Build history of the part. All positions in model axes, mm. A direction names the side the tool comes from. Round coordinates to 2 decimals unless told otherwise and drop trailing zeros. Write each loop counter-clockwise with the first axis right and the second up, starting at its lowest first coordinate (ties: lowest second). Pieces come first, ordered by that corner, then holes. Notation, with made-up numbers: M -9,60 L 14,60 A25 cw 14,96 Z; hole C -13,16 d7. An arc over 180 degrees is marked long. Write item = value, one per line.
from build123d import *

# Parameters (mm, degrees)
SKETCH1_R           = 1.7
BOSS_EXTRUDE1_DEPTH = 5
CUT_EXTRUDE1_DEPTH  = 2
SKETCH3_R           = 3
CUT_EXTRUDE2_DEPTH  = 2
SKETCH4_R           = 1.9
CUT_EXTRUDE3_DEPTH  = 3
SKETCH5_R           = 0.8
CUT_EXTRUDE4_DEPTH  = 3
CUT_EXTRUDE8_DEPTH  = 0.8
FILLET1_R           = 1.5875
CUT_EXTRUDE9_REACH  = 64.803
SKETCH8_W           = 7.193942136
SKETCH8_H           = 8.27
FILLET2_R           = 1.5875
SKETCH9_W           = 5
SKETCH9_H           = 0.25
CUT_EXTRUDE11_DEPTH = 5


with BuildPart() as part:
    # Sketch1 → Boss-Extrude1 (new body)
    with BuildSketch(Plane.XY):
        with BuildLine():
            Line((43, -3.052490593), (43, 3.052490593))
            ThreePointArc((43, 3.052490593), (42.8123201, 3.635702437), (42.319727891, 4))
            ThreePointArc((42.319727891, 4), (39.191767362, 6.313289526), (38, 10.016684732))
            Line((38, 10.016684732), (38, 24.575474703))
            ThreePointArc((38, 24.575474703), (38.684894673, 27.444112294), (40.591836735, 29.693942136))
            ThreePointArc((40.591836735, 29.693942136), (40.892142571, 30.048246049), (41, 30.5))
            Line((41, 30.5), (41, 35.5))
            Line((41, 35.5), (34, 35.5))
            ThreePointArc((34, 35.5), (33.292893219, 35.792893219), (33, 36.5))
            Line((33, 36.5), (33, 43.5))
            Line((33, 43.5), (28, 43.5))
            ThreePointArc((28, 43.5), (27.548246049, 43.392142571), (27.193942136, 43.091836735))
            ThreePointArc((27.193942136, 43.091836735), (24.944112294, 41.184894673), (22.075474703, 40.5))
            Line((22.075474703, 40.5), (10.016684732, 40.5))
            ThreePointArc((10.016684732, 40.5), (6.313289526, 41.691767362), (4, 44.819727891))
            ThreePointArc((4, 44.819727891), (3.635702437, 45.3123201), (3.052490593, 45.5))
            Line((3.052490593, 45.5), (-3.052490593, 45.5))
            ThreePointArc((-3.052490593, 45.5), (-3.635702437, 45.3123201), (-4, 44.819727891))
            ThreePointArc((-4, 44.819727891), (-6.313289526, 41.691767362), (-10.016684732, 40.5))
            Line((-10.016684732, 40.5), (-27.881532566, 40.5))
            ThreePointArc((-27.881532566, 40.5), (-30.750170158, 41.184894673), (-33, 43.091836735))
            ThreePointArc((-33, 43.091836735), (-33.354303912, 43.392142571), (-33.806057864, 43.5))
            Line((-33.806057864, 43.5), (-40, 43.5))
            ThreePointArc((-40, 43.5), (-40.707106781, 43.207106781), (-41, 42.5))
            Line((-41, 42.5), (-41, 36.306057864))
            ThreePointArc((-41, 36.306057864), (-40.892142571, 35.854303912), (-40.591836735, 35.5))
            ThreePointArc((-40.591836735, 35.5), (-38.684894673, 33.250170158), (-38, 30.381532566))
            Line((-38, 30.381532566), (-38, 10.016684732))
            ThreePointArc((-38, 10.016684732), (-39.191767362, 6.313289526), (-42.319727891, 4))
            ThreePointArc((-42.319727891, 4), (-42.8123201, 3.635702437), (-43, 3.052490593))
            Line((-43, 3.052490593), (-43, -3.052490593))
            ThreePointArc((-43, -3.052490593), (-42.8123201, -3.635702437), (-42.319727891, -4))
            ThreePointArc((-42.319727891, -4), (-39.191767362, -6.313289526), (-38, -10.016684732))
            Line((-38, -10.016684732), (-38, -30.381532566))
            ThreePointArc((-38, -30.381532566), (-38.684894673, -33.250170158), (-40.591836735, -35.5))
            ThreePointArc((-40.591836735, -35.5), (-40.892142571, -35.854303912), (-41, -36.306057864))
            Line((-41, -36.306057864), (-41, -42.5))
            ThreePointArc((-41, -42.5), (-40.707106781, -43.207106781), (-40, -43.5))
            Line((-40, -43.5), (-33.806057864, -43.5))
            ThreePointArc((-33.806057864, -43.5), (-33.354303912, -43.392142571), (-33, -43.091836735))
            ThreePointArc((-33, -43.091836735), (-30.750170158, -41.184894673), (-27.881532566, -40.5))
            Line((-27.881532566, -40.5), (-10.016684732, -40.5))
            ThreePointArc((-10.016684732, -40.5), (-6.313289526, -41.691767362), (-4, -44.819727891))
            ThreePointArc((-4, -44.819727891), (-3.635702437, -45.3123201), (-3.052490593, -45.5))
            Line((-3.052490593, -45.5), (3.052490593, -45.5))
            ThreePointArc((3.052490593, -45.5), (3.635702437, -45.3123201), (4, -44.819727891))
            ThreePointArc((4, -44.819727891), (6.313289526, -41.691767362), (10.016684732, -40.5))
            Line((10.016684732, -40.5), (27.881532566, -40.5))
            ThreePointArc((27.881532566, -40.5), (30.750170158, -41.184894673), (33, -43.091836735))
            ThreePointArc((33, -43.091836735), (33.354303912, -43.392142571), (33.806057864, -43.5))
            Line((33.806057864, -43.5), (40, -43.5))
            ThreePointArc((40, -43.5), (40.707106781, -43.207106781), (41, -42.5))
            Line((41, -42.5), (41, -36.306057864))
            ThreePointArc((41, -36.306057864), (40.892142571, -35.854303912), (40.591836735, -35.5))
            ThreePointArc((40.591836735, -35.5), (38.684894673, -33.250170158), (38, -30.381532566))
            Line((38, -30.381532566), (38, -10.016684732))
            ThreePointArc((38, -10.016684732), (39.191767362, -6.313289526), (42.319727891, -4))
            ThreePointArc((42.319727891, -4), (42.8123201, -3.635702437), (43, -3.052490593))
        make_face()
        with Locations((0, -42.5)):
            Circle(SKETCH1_R, mode=Mode.SUBTRACT)
        with Locations((-40, 0)):
            Circle(SKETCH1_R, mode=Mode.SUBTRACT)
        with Locations((40, 0)):
            Circle(SKETCH1_R, mode=Mode.SUBTRACT)
        with Locations((0, 42.5)):
            Circle(SKETCH1_R, mode=Mode.SUBTRACT)
        with Locations((38, 32.5)):
            Circle(SKETCH1_R, mode=Mode.SUBTRACT)
        with Locations((30, 40.5)):
            Circle(SKETCH1_R, mode=Mode.SUBTRACT)
    extrude(amount=-BOSS_EXTRUDE1_DEPTH)

    # Sketch2 → Cut-Extrude1 (cut)
    with BuildSketch(Plane(origin=(0, 0, -5), x_dir=(-1, 0, 0), z_dir=(0, 0, -1))):
        with BuildLine():
            Line((-20, 37.5), (20, 37.5))
            ThreePointArc((20, 37.5), (30.606601718, 33.106601718), (35, 22.5))
            Line((35, 22.5), (35, -22.5))
            ThreePointArc((35, -22.5), (30.606601718, -33.106601718), (20, -37.5))
            Line((20, -37.5), (-20, -37.5))
            ThreePointArc((-20, -37.5), (-30.606601718, -33.106601718), (-35, -22.5))
            Line((-35, -22.5), (-35, 22.5))
            ThreePointArc((-35, 22.5), (-30.606601718, 33.106601718), (-20, 37.5))
        make_face()
    extrude(amount=-CUT_EXTRUDE1_DEPTH, mode=Mode.SUBTRACT)

    # Sketch3 → Cut-Extrude2 (cut)
    with BuildSketch(Plane.XY):
        with Locations((-37, 39.5)):
            Circle(SKETCH3_R)
        with Locations((-37, -39.5)):
            Circle(SKETCH3_R)
        with Locations((37, -39.5)):
            Circle(SKETCH3_R)
        with BuildLine():
            Line((40, 3), (43, 3))
            Line((43, 3), (43, -3))
            Line((43, -3), (40, -3))
            ThreePointArc((40, -3), (37, 0), (40, 3))
        make_face()
        with BuildLine():
            Line((-40, 3), (-43, 3))
            Line((-43, 3), (-43, -3))
            Line((-43, -3), (-40, -3))
            ThreePointArc((-40, -3), (-37, 0), (-40, 3))
        make_face()
        with BuildLine():
            Line((-3, 42.5), (-3, 45.5))
            Line((-3, 45.5), (3, 45.5))
            Line((3, 45.5), (3, 42.5))
            ThreePointArc((3, 42.5), (0, 39.5), (-3, 42.5))
        make_face()
        with BuildLine():
            Line((-3, -42.5), (-3, -45.5))
            Line((-3, -45.5), (3, -45.5))
            Line((3, -45.5), (3, -42.5))
            ThreePointArc((3, -42.5), (0, -39.5), (-3, -42.5))
        make_face()
        with BuildLine():
            Line((38, 29.5), (40.341066152, 29.5))
            ThreePointArc((40.341066152, 29.5), (40.465240963, 29.598536241), (40.591836735, 29.693942136))
            ThreePointArc((40.591836735, 29.693942136), (40.892142571, 30.048246049), (41, 30.5))
            Line((41, 30.5), (41, 35.5))
            Line((41, 35.5), (35, 35.5))
            Line((35, 35.5), (35, 32.5))
            ThreePointArc((35, 32.5), (35.878679656, 30.378679656), (38, 29.5))
        make_face()
        with BuildLine():
            Line((30, 37.5), (33, 37.5))
            Line((33, 37.5), (33, 43.5))
            Line((33, 43.5), (28, 43.5))
            ThreePointArc((28, 43.5), (27.548246049, 43.392142571), (27.193942136, 43.091836735))
            ThreePointArc((27.193942136, 43.091836735), (27.098536241, 42.965240963), (27, 42.841066152))
            Line((27, 42.841066152), (27, 40.5))
            ThreePointArc((27, 40.5), (27.878679656, 38.378679656), (30, 37.5))
        make_face()
    extrude(amount=-CUT_EXTRUDE2_DEPTH, mode=Mode.SUBTRACT)

    # Sketch4 → Cut-Extrude3 (cut)
    with BuildSketch(Plane.XY.offset(-2)):
        with Locations((-37, 39.5)):
            Circle(SKETCH4_R)
        with Locations((37, -39.5)):
            Circle(SKETCH4_R)
        with Locations((-37, -39.5)):
            Circle(SKETCH4_R)
    extrude(amount=-CUT_EXTRUDE3_DEPTH, mode=Mode.SUBTRACT)

    # Sketch5 → Cut-Extrude4 (cut)
    with BuildSketch(Plane.XY):
        with Locations((-17.109, -19.609)):
            Circle(SKETCH5_R)
        with Locations((-14.109, -19.609)):
            Circle(SKETCH5_R)
        with Locations((-11.109, -19.609)):
            Circle(SKETCH5_R)
        with Locations((-8.109, -19.609)):
            Circle(SKETCH5_R)
        with Locations((-17.109, -22.609)):
            Circle(SKETCH5_R)
        with Locations((-14.109, -22.609)):
            Circle(SKETCH5_R)
        with Locations((-11.109, -22.609)):
            Circle(SKETCH5_R)
        with Locations((-8.109, -22.609)):
            Circle(SKETCH5_R)
        with Locations((-17.109, -25.609)):
            Circle(SKETCH5_R)
        with Locations((-14.109, -25.609)):
            Circle(SKETCH5_R)
        with Locations((-11.109, -25.609)):
            Circle(SKETCH5_R)
        with Locations((-8.109, -25.609)):
            Circle(SKETCH5_R)
        with Locations((-17.109, -16.609)):
            Circle(SKETCH5_R)
        with Locations((-14.109, -16.609)):
            Circle(SKETCH5_R)
        with Locations((-11.109, -16.609)):
            Circle(SKETCH5_R)
        with Locations((-8.109, -16.609)):
            Circle(SKETCH5_R)
    extrude(amount=-CUT_EXTRUDE4_DEPTH, mode=Mode.SUBTRACT)

    # Sketch7 → Cut-Extrude8 (cut)
    with BuildSketch(Plane.XY):
        with BuildLine():
            Line((22.4125, 38.73), (-34.100500043, 38.73))
            ThreePointArc((-34.100500043, 38.73), (-35.171065884, 37.12197561), (-37, 36.5))
            Line((-37, 36.5), (-37, 35.23))
            Line((-37, 35.23), (22.4125, 35.23))
            ThreePointArc((22.4125, 35.23), (23.535032015, 35.694967985), (24, 36.8175))
            Line((24, 36.8175), (24, 37.1425))
            ThreePointArc((24, 37.1425), (23.535032015, 38.265032015), (22.4125, 38.73))
        make_face()
    extrude(amount=-CUT_EXTRUDE8_DEPTH, mode=Mode.SUBTRACT)

    # Fillet1
    # the kernel refuses this fillet: 1.5875 mm, written as the material it adds along each edge
    with BuildSketch(Plane(origin=(-37, 35.23, 0), x_dir=(1.4714388937389554e-12, 1.0, 0), z_dir=(0, 0, -1))) as fillet1_piece_1:
        with BuildLine():
            CenterArc((1.5875, 1.555425987), FILLET1_R, 180, 78.463040967)
            Line((0, 1.555425987), (-0.03175, 1.555425987))
            Line((-0.03175, 1.555425987), (-0.03175, 0))
            Line((-0.03175, 0), (0, -0.03175))
            ThreePointArc((0, -0.03175), (0.635, -0.03175), (1.26365, -0.03110852))
            Line((1.26365, -0.03110852), (1.27, 0))
        make_face()
    extrude(amount=4.688564967)

    # Cut-Extrude9: up to this face of the body (flat: up to its plane)
    cut_extrude9_end = Plane(part.part.faces().sort_by_distance((-39.915147186, 39.5, -2))[0])
    # Sketch8 → Cut-Extrude9 (cut, up to the picked face)
    with BuildSketch(Plane.XY, mode=Mode.PRIVATE) as cut_extrude9_sk1:
        with Locations((-37.403028932, 39.365)):
            Rectangle(SKETCH8_W, SKETCH8_H)
    cut_extrude9_tool1 = split(extrude(cut_extrude9_sk1.sketch, amount=-CUT_EXTRUDE9_REACH, mode=Mode.PRIVATE), bisect_by=cut_extrude9_end, keep=Keep.BOTH, mode=Mode.PRIVATE)
    add(cut_extrude9_tool1.solids().sort_by(Axis((-37.403029, 39.365, 0), (0, 0, -1)))[0], mode=Mode.SUBTRACT)

    # Fillet2
    fillet2_edges = [part.edges().sort_by_distance(p)[0] for p in [
        (-33.806057864, 35.23, -1.4),
    ]]
    fillet(fillet2_edges, radius=FILLET2_R)

    # Sketch9 → Cut-Extrude11 (cut, symmetric)
    with BuildSketch(Plane(origin=(0, 0, 0), x_dir=(0, 0, -1), z_dir=(1, 0, 0))):
        with Locations((2.5, 45.375)):
            Rectangle(SKETCH9_W, SKETCH9_H)
    extrude(amount=CUT_EXTRUDE11_DEPTH, both=True, mode=Mode.SUBTRACT)


solid = part.part
1. Tool access for faces 1 (the face through (31.3, 41.9, -2)), 2 (the face through (0.1, 39.5, -1)), 3 (the face through (-37, -43.5, -2)): list every direction of +Z, -Z, +X, -X, +Y, -Y with a clear straight run to the whole face (end or side of a thin tool).
Responses:
face_1 = +Z, +X, +Y
face_2 = +Z, +Y
face_3 = +Z, -Z, -X, -Y
2. Mould opens along Y. For faces 4 (the face through (35, 34, -1)), 5 (the face through (-30.49, 33.22, -4.01)), 6 (the face through (35.86, 30.4, -0.99)), 7 (the face through (-39.21, -37.47, -0.99)) say: pulls with the +Y half, pulls with the -Y half, needs draft (parallel to the pull), parting line crosses it, or undercut.
Responses:
face_4 = needs draft
face_5 = undercut
face_6 = pulls with the +Y half
face_7 = undercut
3. Band-saw the part on B-B (y = -9). List the corners of the cut face in (x, z), plus the area to 3 significant figures.
Responses:
outline = M -38.08,-5 L -35,-5 L -35,-3 L 35,-3 L 35,-5 L 38.08,-5 L 38.08,0 L -38.08,0 Z
area = 241 mm²
4. Band-saw the part on A-A (x = 0). List the corners of the cut face in (y, z).
Responses:
outline = M -45.5,-5 L -44.2,-5 L -44.2,-2 L -45.5,-2 Z; M -40.8,-5 L -37.5,-5 L -37.5,-3 L 37.5,-3 L 37.5,-5 L 40.8,-5 L 40.8,-2 L 39.5,-2 L 39.5,0 L 38.73,0 L 38.73,-0.8 L 35.23,-0.8 L 35.23,0 L -39.5,0 L -39.5,-2 L -40.8,-2 Z; M 44.2,-5 L 45.25,-5 L 45.25,-2 L 44.2,-2 Z
5. Probe probe 1 along Y at (x, z) = (-37, -2.9); probe 2 along X at (y, z) = (1.5, -4.05); probe 3 along X at (y, z) = (-16.5, -1.1). List the from-to ranges inside material, lowest first.
Responses:
probe_1 = -43.5 to -41.4, -37.6 to 37.6, 41.4 to 43.5
probe_2 = -43 to -40.8, -39.2 to -35, 35 to 39.2, 40.8 to 43
probe_3 = -38 to -17.9, -16.32 to -14.9, -13.32 to -11.9, -10.32 to -8.9, -7.32 to 38
6. Flat gauge pins, fed straight in: pin 1 (1 mm diameter, centred on x = 42, z = -1.5, fed in from -Y); pin 2 (1 mm diameter, centred on x = 10, z = -3.5, fed in from +Y); pin 3 (1 mm diameter, centred on x = 26, z = -3.5, fed in from +Y). Where does each tip first touch, or does it go through?
Responses:
pin_1 = -4.34
pin_2 = 40.52
pin_3 = 42.3
7. Band-saw the part on C-C (y = -33). List the corners of the cut face in (x, z) (3 decimals), plus the area to 3 significant figures.
Responses:
outline = M -38.565,-5 L -30.712,-5 L -30.712,-3 L 30.712,-3 L 30.712,-5 L 38.565,-5 L 38.565,0 L -38.565,0 Z
area = 263 mm²
